Design review of the part built by this model. Coordinates are the model's own, in mm. Face numbers are marked on the shaded views. Round coordinates to 2 decimals unless told otherwise and drop trailing zeros. Order: outer loops, then holes, each group sorted by start corner. A loop starts at its lowest first (then second) coordinate and runs counter-clockwise, first axis right, second up. Notation, with made-up numbers: (80.5, -32.75) - (139.5, -32.75) arc R17 ccw to (139.5, -4.75) - close; hole circle Ø1 at (67.5, 55). An arc over 180 degrees is marked (long way). Use CSV: the item, a comma, the result in double quotes.
from build123d import *

# Parameters (mm, degrees)
SKETCH2_W           = 55
SKETCH2_H           = 24
SKETCH2_R           = 4
SKETCH2_R_2         = 1.5
BOSS_EXTRUDE1_DEPTH = 2
SKETCH5_R           = 2.5
SKETCH5_R_2         = 1.5
BOSS_EXTRUDE2_DEPTH = 2
FILLET1_R           = 2.5


with BuildPart() as part:
    # Sketch2 → Boss-Extrude1 (new body)
    with BuildSketch(Plane(origin=(0, 0, 0), x_dir=(1, 0, 0), z_dir=(0, 1, 0))):
        Rectangle(SKETCH2_W, SKETCH2_H)
        Circle(SKETCH2_R, mode=Mode.SUBTRACT)
        with Locations((0, 7)):
            Circle(SKETCH2_R_2, mode=Mode.SUBTRACT)
        with Locations((7, 0)):
            Circle(SKETCH2_R_2, mode=Mode.SUBTRACT)
        with Locations((0, -7)):
            Circle(SKETCH2_R_2, mode=Mode.SUBTRACT)
        with Locations((-7, 0)):
            Circle(SKETCH2_R_2, mode=Mode.SUBTRACT)
        with Locations((-18.6, 0)):
            Circle(SKETCH2_R_2, mode=Mode.SUBTRACT)
        with Locations((18.6, 0)):
            Circle(SKETCH2_R_2, mode=Mode.SUBTRACT)
    extrude(amount=BOSS_EXTRUDE1_DEPTH)

    # Sketch5 → Boss-Extrude2 (add)
    with BuildSketch(Plane.ZY.offset(27.5)):
        with BuildLine():
            Line((12, 0), (12, 52))
            ThreePointArc((12, 52), (0, 64), (-12, 52))
            Line((-12, 52), (-12, 0))
            Line((-12, 0), (12, 0))
        make_face()
        with Locations((0, 52)):
            Circle(SKETCH5_R, mode=Mode.SUBTRACT)
        with Locations((0, 59)):
            Circle(SKETCH5_R_2, mode=Mode.SUBTRACT)
        with Locations((7, 52)):
            Circle(SKETCH5_R_2, mode=Mode.SUBTRACT)
        with Locations((0, 45)):
            Circle(SKETCH5_R_2, mode=Mode.SUBTRACT)
        with Locations((-7, 52)):
            Circle(SKETCH5_R_2, mode=Mode.SUBTRACT)
        with Locations((0, 33.4)):
            Circle(SKETCH5_R_2, mode=Mode.SUBTRACT)
        with Locations((0, 16.5)):
            Circle(SKETCH5_R_2, mode=Mode.SUBTRACT)
    boss_extrude2 = extrude(amount=-BOSS_EXTRUDE2_DEPTH)

    # Mirror1: Boss-Extrude2 across plane
    add(boss_extrude2.mirror(Plane(origin=(0, 0, 0), x_dir=(0, 0, 1), z_dir=(1, 0, 0))))

    # Fillet1
    fillet1_edges = [part.edges().sort_by_distance(p)[0] for p in [
        (-27.5, 0, 0),
        (27.5, 0, 0),
    ]]
    fillet(fillet1_edges, radius=FILLET1_R)


solid = part.part
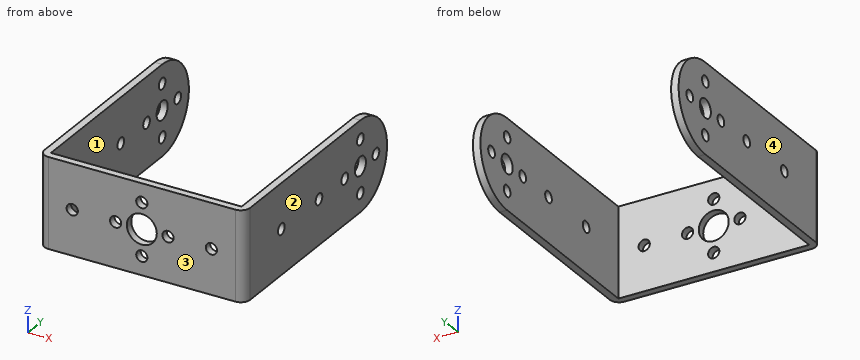
1) The part is to be moulded in two halves that separate along X. For the marked faces 1, 2, 3 and 4, say which applies: +X half, -X half, draft (parallel to the pull), parting line (faces both ways), or undercut.
Data:
face 1,"undercut"
face 2,"+X half"
face 3,"draft"
face 4,"-X half"
2) We need section C-C (z = 0). Give the number of separate pieces and of enclosed holes in the cut face, then the cut area to 3 significant figures.
Data:
separate pieces,"16"
enclosed holes,"0"
area,"247 mm2"
3) To check wall thickness, follow L1, parallel to Z at x = 0, y = 0.65; L2, parallel to X at y = 26, z = 5.75; L3, parallel to Y at x = 15, z = 7.75. State the ranges of each line that lie inside material, in increasing order. Write a range as from..to.
Data:
L1,"z = -12..-8.5, -5.5..-4, 4..5.5, 8.5..12"
L2,"x = -27.5..-25.5, 25.5..27.5"
L3,"y = 0..2"
4) We need section B-B (x = 18.6). Give the boundary of the cut face in (y, z), then the cut area to 3 significant figures.
Data:
outline,"(0, -12) - (2, -12) - (2, -1.5) - (0, -1.5) - close; (0, 1.5) - (2, 1.5) - (2, 12) - (0, 12) - close"
area,"42.0 mm2"
5) Insertion check: pin 1 Ø3 at (x, z) = (-14.5, 5.5) entering from +Y; pin 2 Ø6.5 at (y, z) = (52, 0) entering from -X. Each pin has a flat end and moves straight along its axis. Give the tip position at first contact, or say it passes through.
Data:
pin 1,"stops at y = 2"
pin 2,"stops at x = -27.5"
6) We need section A-A (y = 45). Give the boundary of the cut face in (x, z).
Data:
outline,"(-27.5, -12) - (-25.5, -12) - (-25.5, -1.5) - (-27.5, -1.5) - close; (-27.5, 1.5) - (-25.5, 1.5) - (-25.5, 12) - (-27.5, 12) - close; (25.5, -12) - (27.5, -12) - (27.5, -1.5) - (25.5, -1.5) - close; (25.5, 1.5) - (27.5, 1.5) - (27.5, 12) - (25.5, 12) - close"
7) We need section D-D (y = 59). Give the boundary of the cut face in (x, z).
Data:
outline,"(-27.5, -9.75) - (-25.5, -9.75) - (-25.5, -1.5) - (-27.5, -1.5) - close; (-27.5, 1.5) - (-25.5, 1.5) - (-25.5, 9.75) - (-27.5, 9.75) - close; (25.5, -9.75) - (27.5, -9.75) - (27.5, -1.5) - (25.5, -1.5) - close; (25.5, 1.5) - (27.5, 1.5) - (27.5, 9.75) - (25.5, 9.75) - close"
